Autodesk Inventor part; units mm, degrees
ref_plane "YZ Plane" through (0, 0, 0) normal (1, 0, 0) x (0, 1, 0)
ref_plane "XZ Plane" through (0, 0, 0) normal (0, 1, 0) x (-1, 0, 0)
ref_plane "XY Plane" through (0, 0, 0) normal (0, 0, 1) x (1, 0, 0)
sketch "Эскиз1" plane through (0, 0, 0) normal (0, 1, 0) x (-1, 0, 0)
  line L0 (0, 0) -> (46, 0)
  line L1 (46, 0) -> (46, -25)
  line L2 (46, -25) -> (0, -25)
  line L3 (0, -25) -> (0, 0)
  circle A0 centre (10.8656, -11.5046) radius 8
  circle A1 centre (10.8656, -11.5046) radius 9.25
  dimension "d0" = 25
  dimension "d1" = 46
  dimension "d2" = 16
  dimension "d3" = 18.5
extrude "Выдавливание1" add sketch "Эскиз1" along normal blind 8 contours L0 L1 L2 L3 | A1
extrude "Выдавливание2" cut sketch "Эскиз1" along normal blind 1 contours A1
sketch "Эскиз2" plane through (-46, 0, -25) normal (-1, 0, 0) x (0, 0, 1)
  line L0 (0, 0) -> (0, 8)
  line L1 (0, 4) -> (25, 4) construction
  line L2 (25, 0) -> (25, 8)
  circle A0 centre (13.1, 4) radius 2
  dimension "d8" = 4
  dimension "d15" = 13.1
sketch "Эскиз3" plane through (0, 0, -25) normal (0, 0, -1) x (-1, 0, 0)
  line L0 (46, 0) -> (46, 8)
  line L1 (46, 4) -> (17.4, 4)
  circle A0 centre (17.4, 4) radius 2
  point P0 (0, 0)
  dimension "d9" = 4
  dimension "d14" = 28.6
extrude "Выдавливание3" cut sketch "Эскиз3" against normal blind 5
extrude "Выдавливание4" cut sketch "Эскиз2" against normal blind 5
fillet "Сопряжение1" radius 0.5 6 edges at (0, 0, -12.5) (0, 8, -12.5) (0, 4, 0) (0, 4, -25) (-23, 8, 0) (-23, 0, 0)
fillet "Сопряжение2" radius 0.5 1 edges at (-2.8656, 8, -11.5046)
properties part number "держатель шкивов 2"
Design review of the part built by this model. Coordinates are the model's own, in mm. A direction names the side the tool comes from. Coordinates: 2 decimals unless noted, no trailing zeros. Loops run counter-clockwise (first coordinate to the right, second up) from the corner with the lowest first, then second, coordinate; pieces in that order, holes last. Notation, with made-up numbers: (2, 84.25) -> (61, 84.25) arc R29 ccw to (61, 120.25) -> close; hole circle Ø11 at (83.25, 56). An arc over 180 degrees is marked (long way). Use a Markdown table: item, result. Add a question column.
Item 1: We need section B-B, the plane y = 5.5. Write out the cut boundary in (x, z).
Item 2: We need section A-A, the plane z = -22.5. Write out the cut boundary in (x, y).
Item 3: The part is to be moulded in two halves that separate along Y. For faces 1 (the cylindrical face through (-8.86, 0.493, -2.475)), 2 (the cylindrical face through (-43.5, 2.8, -13.5)), 3 (the flat face through (-28, 8, -13)), 4 (the flat face through (-28, 0, -13)), say which applies: +Y half, -Y half, draft (parallel to the pull), parting line (faces both ways), or undercut.
Item 4: Clearance check with flat-ended pins moving along their axes: P1, Ø10, axis at x = -6.5, z = -18, coming from the +Y side; P2, Ø2, axis at x = -18, y = 3.5, coming from the -Z side. State where each tip first meets the part, or that it passes through.
Item 5: Machinability: for faces 5 (the flat face through (-23, 4, 0)), 6 (the flat face through (-4, 1, -16)), 7 (the flat face through (-41, 4, -12)), 8 (the flat face through (-17, 4, -20)), which of the approach directions +Z, -Z, +X, -X, +Y, -Y give a long, thin tool a straight path to every point of the face, cutting with its end or side? Answer none if there is none.
Item 6: Wall thickness on L1, parallel to Y at x = -17.4, z = -23.1; L2, parallel to X at y = 4, z = -13.5; L3, parallel to X at y = 1.5, z = -17: over which ranges is each line inside the solid? List them lowest first. Write a range as from..to.
Numbers:
| question | item | result |
|---|---|---|
| 1 | outline | (-46, -25) -> (-18.72, -25) -> (-18.72, -20) -> (-16.08, -20) -> (-16.08, -25) -> (-0.5, -25) arc R0.5 ccw to (0, -24.5) -> (0, -0.5) arc R0.5 ccw to (-0.5, 0) -> (-46, 0) -> (-46, -10.58) -> (-41, -10.58) -> (-41, -13.22) -> (-46, -13.22) -> close; hole circle Ø16 at (-10.87, -11.5) |
| 2 | outline | (-46, 0) -> (-0.5, 0) arc R0.5 ccw to (0, 0.5) -> (0, 7.5) arc R0.5 ccw to (-0.5, 8) -> (-46, 8) -> close; hole circle Ø4 at (-17.4, 4) |
| 3 | face 1 | draft |
| 3 | face 2 | undercut |
| 3 | face 3 | +Y half |
| 3 | face 4 | -Y half |
| 4 | P1 | stops at y = 8 |
| 4 | P2 | stops at z = -20 |
| 5 | face 5 | +Z, +X, -X, +Y, -Y |
| 5 | face 6 | -Y |
| 5 | face 7 | -X |
| 5 | face 8 | -Z |
| 6 | L1 | y = 0..2, 6..8 |
| 6 | L2 | x = -41..-18.61, -3.12..0 |
| 6 | L3 | x = -46..-16.68, -5.05..0 |
